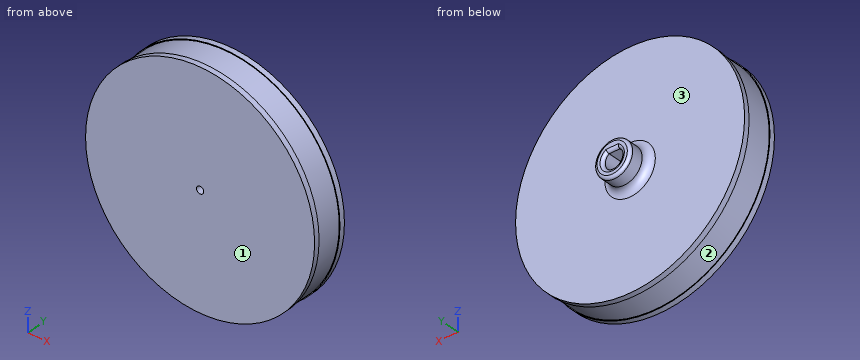
Autodesk Fusion 360 part; units mm, degrees
sketch "spodek" plane through (0, 0, 0) normal (0, 1, 0) x (1, 0, 0)
  circle A0 centre (0, 0) radius 31.75
  circle A1 centre (0, 0) radius 1
  dimension "d1" = 63.5
  dimension "d2" = 2
extrude "Extrude1" add sketch "spodek" along normal blind 1.5
sketch "prostredek" plane through (0, 1.5, 0) normal (0, 1, 0) x (-1, 0, 0)
  circle A0 centre (0, 0) radius 1
  circle A1 centre (0, 0) radius 31.75
  circle A2 centre (0, 0) radius 31.55
  line L0 (3.493, -6.05) -> (6.9859, 0)
  line L1 (6.9859, 0) -> (3.493, 6.05)
  line L2 (3.493, 6.05) -> (-3.493, 6.05)
  line L3 (-3.493, 6.05) -> (-6.9859, 0)
  line L4 (-6.9859, 0) -> (-3.493, -6.05)
  line L5 (-3.493, -6.05) -> (3.493, -6.05)
  dimension "d5" = -0.2
  dimension "d6" = 6.05
extrude "Extrude2" add sketch "prostredek" along normal blind 7 contours A2 | L0 L1 L2 L3 L4 L5
sketch "Sketch3" plane through (0, 8.5, 0) normal (0, 1, 0) x (-1, 0, 0)
  circle A0 centre (0, 0) radius 31.75
  line L0 (-1.4902, 2.1) -> (1.4902, 2.1)
  arc A1 (-1.4902, 2.1) -> (1.4902, 2.1) centre (0, 0) ccw
  dimension "d12" = 5.15
  dimension "d13" = 2.1
extrude "Extrude4" cut sketch "Sketch3" against normal blind 6 contours L0 A1
extrude "Extrude5" add sketch "Sketch3" along normal blind 1.5
sketch "Sketch4" plane through (0, 10, 0) normal (0, 1, 0) x (-1, 0, 0)
  arc A0 (-1.4902, 2.1) -> (1.4902, 2.1) centre (0, 0) ccw
  line L0 (-1.4902, 2.1) -> (1.4902, 2.1)
  circle A1 centre (0, 0) radius 31.75
  circle A2 centre (0, 0) radius 5
  dimension "d22" = 10
extrude "Extrude6" add sketch "Sketch4" along normal blind 6 contours A2
fillet "Fillet3" radius 0.8 1 faces at (-0.1246, 16, 3.062)
fillet "Fillet4" radius 2 1 edges at (4.6616, 10, 1.8081)
Can you work these out from the model? Positions are in its coordinate system, mm. Face numbers are marked on the shaded views. Round coordinates to 2 decimals unless told otherwise and drop trailing zeros. Order: outer loops, then holes, each group sorted by start corner. A loop starts at its lowest first (then second) coordinate and runs counter-clockwise, first axis right, second up.
(1) If we section it at D-D (x = -12): Please give me the cut outline in (y, z).
Results are:
outline: (0, -29.39) - (1.5, -29.39) - (1.5, -29.18) - (8.5, -29.18) - (8.5, -29.39) - (10, -29.39) - (10, 29.39) - (8.5, 29.39) - (8.5, 29.18) - (1.5, 29.18) - (1.5, 29.39) - (0, 29.39) - close
(2) If I drill on L1, parallel to Z at x = 0, y = 7; L2, parallel to X at y = 1.35, z = 0; L3, parallel to Y at x = -24.5, z = 15, over which ranges is the centre line in solid material (lowest first)?
Results are:
L1: z = -31.55 to -2.58, 2.1 to 31.55
L2: x = -31.75 to -1, 1 to 31.75
L3: y = 0 to 10
(3) We'd pull the mould along Y, two halves only. Please class the marked faces 1, 2 and 3: +Y half, -Y half, draft (parallel to the pull), parting line (faces both ways), or undercut.
Results are:
face 1: -Y half
face 2: undercut
face 3: +Y half
(4) If we section it at C-C (z = 18.5): Please give me the cut outline in (x, y), plus the area to 3 significant figures.
Results are:
outline: (-25.8, 0) - (25.8, 0) - (25.8, 1.5) - (25.56, 1.5) - (25.56, 8.5) - (25.8, 8.5) - (25.8, 10) - (-25.8, 10) - (-25.8, 8.5) - (-25.56, 8.5) - (-25.56, 1.5) - (-25.8, 1.5) - close
area: 513 mm2
(5) If we section it at B-B (y = 14): Please give me the cut outline in (x, z).
Results are:
outline: circle Ø10 at (0, 0); hole (-1.49, 2.1) arc R2.58 ccw (long way) to (1.49, 2.1) - close
(6) I'm going to push flat-ended pins straight in: pin 1 (2.5 mm diameter, centred on x = -0.5, y = 11, fed in from -Z); pin 2 (4.5 mm diameter, centred on x = 0, z = 0, fed in from -Y); pin 3 (19 mm diameter, centred on x = 3, z = -14.5, fed in from +Y); pin 4 (5 mm diameter, centred on y = 10, z = -8.5, fed in from +X). Where does each tip first touch, or does it pass through?
Results are:
pin 1: stops at z = -31.75
pin 2: stops at y = 0
pin 3: stops at y = 10.94
pin 4: stops at x = 31.18
